Could you check a few things on this model? Use its own coordinates, in mm. Give positions to 0.01 mm unless a question says otherwise; leave off trailing zeros. Loops run counter-clockwise (first coordinate to the right, second up) from the corner with the lowest first, then second, coordinate; pieces in that order, holes last. Notation, with made-up numbers: (73.25, -19) - (91.25, -19) arc R12 cw to (91.25, -5) - close; hole circle Ø3 at (-36.5, 81). An arc over 180 degrees is marked (long way). Use CSV: the item, a comma, the result in double quotes.
Autodesk Inventor part; units mm, degrees
ref_plane "YZ Plane" through (0, 0, 0) normal (1, 0, 0) x (0, 1, 0)
ref_plane "XZ Plane" through (0, 0, 0) normal (0, 1, 0) x (-1, 0, 0)
ref_plane "XY Plane" through (0, 0, 0) normal (0, 0, 1) x (1, 0, 0)
sketch "Boceto1" plane through (0, 0, 0) normal (0, 0, 1) x (1, 0, 0)
  line L0 (112.2616, 170.6474) -> (112.2616, 129.3648)
  arc A0 (112.2616, 129.3648) -> (118.4288, 114.4759) centre (133.3177, 129.3648) ccw
  line L1 (118.4288, 114.4759) -> (162.1204, 70.7843)
  arc A1 (166.2045, 60.9244) -> (162.1204, 70.7843) centre (152.2606, 60.9244) ccw
  line L2 (166.2045, 60.9244) -> (166.2045, -74.0436)
  arc A2 (152.2606, -87.9875) -> (166.2045, -74.0436) centre (152.2606, -74.0436) ccw
  line L3 (152.2606, -87.9875) -> (77.1714, -87.9875)
  arc A3 (77.1714, -87.9875) -> (28.3364, -107.4286) centre (77.1714, -159.0436) ccw
  arc A4 (-0.1519, -130.4951) -> (28.3364, -107.4286) centre (-135.1799, 65.3964) ccw
  arc A5 (-56.306, -147.9736) -> (-0.1519, -130.4951) centre (-56.306, -49.0297) ccw
  line L4 (-56.306, -147.9736) -> (-120.6823, -147.9736)
  arc A6 (-139.6262, -129.0297) -> (-120.6823, -147.9736) centre (-120.6823, -129.0297) ccw
  line L5 (-139.6262, -129.0297) -> (-139.6262, 60.9244)
  arc A7 (-135.5422, 70.7843) -> (-139.6262, 60.9244) centre (-125.6823, 60.9244) ccw
  line L6 (-135.5422, 70.7843) -> (-91.7934, 114.533)
  arc A8 (-91.7934, 114.533) -> (-85.6262, 129.4219) centre (-106.6823, 129.4219) ccw
  line L7 (-85.6262, 129.4219) -> (-85.6262, 170.6474)
  line L8 (-85.6262, 170.6474) -> (112.2616, 170.6474)
extrude "Extrusión1" add sketch "Boceto1" along normal blind 2
fillet "Empalme1" radius 2 2 edges at (-85.6262, 170.6474, 1) (112.2616, 170.6474, 1)
sketch "Boceto2" plane through (0, 0, 2) normal (0, 0, 1) x (1, 0, 0)
  line L0 (-139.6262, -129.0297) -> (-139.6262, 60.9244)
  circle A0 centre (-124.6262, 30.7843) radius 1.25
  circle A1 centre (-124.6262, 15.7843) radius 1.25
  circle A2 centre (-124.6262, -92.9736) radius 1.25
  circle A3 centre (-124.6262, -107.9736) radius 1.25
  point P0 (-135.5422, 70.7843)
  point P1 (-120.6823, -147.9736)
  point P2 (0, 0)
  dimension "d3" = 2.5
  dimension "d4" = 2.5
  dimension "d5" = 2.5
  dimension "d6" = 2.5
  dimension "d7" = 15
  dimension "d8" = 15
  dimension "d10" = 40
  dimension "d11" = 15
  dimension "d12" = 15
  dimension "d13" = 40
extrude "Extrusión2" cut sketch "Boceto2" against normal blind 2
sketch "Boceto3" plane through (0, 0, 0) normal (0, 0, -1) x (-1, 0, 0)
  line L0 (-166.2045, 60.9244) -> (-166.2045, -74.0436)
  line L1 (-152.2606, -87.9875) -> (-77.1714, -87.9875)
  circle A0 centre (-151.2045, 32.0125) radius 1.75
  circle A1 centre (-151.2045, -37.9875) radius 1.25
  point P0 (0, 0)
  dimension "d16" = 3.5
  dimension "d17" = 2.5
  dimension "d18" = 70
  dimension "d19" = 50
  dimension "d20" = 15
extrude "Extrusión3" cut sketch "Boceto3" against normal blind 2
properties part number "porta frontal"
1) I need wall thicknesses on line 1 along X through (y, z) = (129, 0.6); line 2 along X through (y, z) = (61, 1.65); line 3 along Y through (x, z) = (98, 0.65). Which ranges of each line are inside material? Lowest first, please.
Answer below:
line 1,"x = -85.63 to 112.26"
line 2,"x = -139.63 to 166.2"
line 3,"y = -87.99 to 170.65"
2) I'm going to push a flat-ended pin straight in: P1, Ø1, axis at y = 143, z = 0.5, coming from the -X side. Where does the tip first touch, or does it pass through?
Answer below:
P1,"stops at x = -85.63"
3) Suppose I cut it at B-B (x = 54.5). Please give me the cut outline in (y, z).
Answer below:
outline,"(-91.7, 0) - (170.65, 0) - (170.65, 2) - (-91.7, 2) - close"
4) Suppose I cut it at A-A (z = 1.15). Please give me the cut outline in (x, y), plus the area to 3 significant figures.
Answer below:
outline,"(-139.63, -129.03) arc R18.94 ccw to (-120.68, -147.97) - (-56.31, -147.97) arc R98.94 ccw to (-0.15, -130.5) arc R237.93 ccw to (28.34, -107.43) arc R71.06 cw to (77.17, -87.99) - (152.26, -87.99) arc R13.94 ccw to (166.2, -74.04) - (166.2, 60.92) arc R13.94 ccw to (162.12, 70.78) - (118.43, 114.48) arc R21.06 cw to (112.26, 129.36) - (112.26, 168.65) arc R2 ccw to (110.26, 170.65) - (-83.63, 170.65) arc R2 ccw to (-85.63, 168.65) - (-85.63, 129.42) arc R21.06 cw to (-91.79, 114.53) - (-135.54, 70.78) arc R13.94 ccw to (-139.63, 60.92) - close; hole circle Ø2.5 at (-124.63, -107.97); hole circle Ø2.5 at (-124.63, -92.97); hole circle Ø2.5 at (-124.63, 15.78); hole circle Ø2.5 at (-124.63, 30.78); hole circle Ø3.5 at (151.2, 32.01); hole circle Ø2.5 at (151.2, -37.99)"
area,"79,900 mm2"
5) Suppose I cut it at C-C (y = -115.5). Please give me the cut outline in (x, z).
Answer below:
outline,"(-139.63, 0) - (19.36, 0) - (19.36, 2) - (-139.63, 2) - close"
